Model file for the job. Use its own axes, mm. Face numbers are marked on the shaded views. A direction names the side the tool comes from. Give positions to 0.01 mm unless a question says otherwise; leave off trailing zeros. Loops run counter-clockwise (first coordinate to the right, second up) from the corner with the lowest first, then second, coordinate; pieces in that order, holes last. Notation, with made-up numbers: (68, -18) - (84, -18) arc R23 ccw to (84, -6) - close; hole circle Ø3 at (-38, 10.5). An arc over 180 degrees is marked (long way). Answer as CSV lines item,"result". Start each with the question number.
Item 1: Tool access for the marked faces 4, 5 and 6: list every direction of +Z, -Z, +X, -X, +Y, -Y with a clear straight run to the whole face (end or side of a thin tool).
Item 2: Pin check, flat tips, straight feed: pin 1 (8 mm diameter, centred on y = 4, z = 10.5, fed in from +X); pin 2 (3.5 mm diameter, centred on y = 2.5, z = 11.5, fed in from -X); pin 3 (3 mm diameter, centred on x = -16.5, y = 0.5, fed in from +Z). Stop position of each tip, or through.
Item 3: Pull direction X, two halves, no side cores. Call the marked faces 1, 2 and 3: pulls with the +X half, pulls with the -X half, needs draft (parallel to the pull), parting line crosses it, or undercut.
Item 4: Saw through at C-C on z = -14.5. Give the cut face in (x, y).
Item 5: Saw through at B-B on y = -4. Give the cut face in (x, z), plus the area to 3 significant figures.
Item 6: Drill centre lines: L1, parallel to X at y = 3.75, z = 0; L2, parallel to X at y = 5.5, z = 13; L3, parallel to X at y = -6, z = -18.5. Where is each one in solid material? Low to high. Write a range as from..to.
Item 7: Saw through at D-D on x = -19. Give the cut face in (y, z).
Item 8: Saw through at A-A on z = 0. Give the cut face in (x, y), plus the area to 3 significant figures.
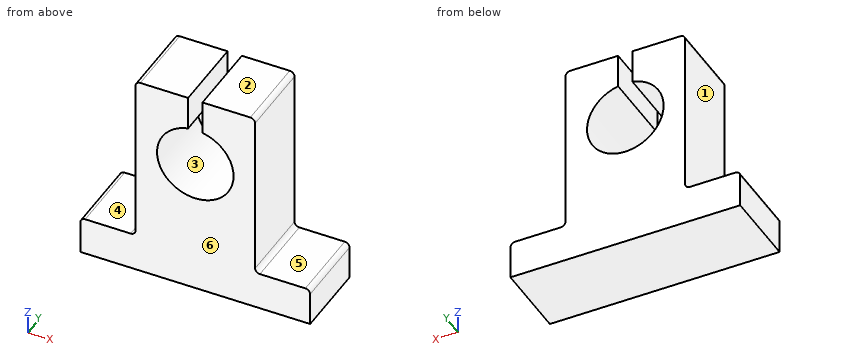
from build123d import *

# Parameters (mm, degrees)
F1_DEPTH = 8


with BuildPart() as f1:
    # F0 (on Front) → F1 (new body, symmetric)
    with BuildSketch(Plane.XZ):
        with BuildLine():
            Line((-24, -29), (24, -29))
            Line((24, -29), (24, -22))
            ThreePointArc((24, -22), (23.707107, -21.292893), (23, -21))
            Line((23, -21), (13.5, -21))
            ThreePointArc((13.5, -21), (12.792893, -20.707107), (12.5, -20))
            Line((12.5, -20), (12.5, 14))
            ThreePointArc((12.5, 14), (12.207107, 14.707107), (11.5, 15))
            Line((11.5, 15), (1.5, 15))
            Line((1.5, 15), (1.5, 7.858117))
            ThreePointArc((1.5, 7.858117), (0, -8), (-1.5, 7.858117))
            Line((-1.5, 7.858117), (-1.5, 15))
            Line((-1.5, 15), (-11.5, 15))
            ThreePointArc((-11.5, 15), (-12.207107, 14.707107), (-12.5, 14))
            Line((-12.5, 14), (-12.5, -20))
            ThreePointArc((-12.5, -20), (-12.792893, -20.707107), (-13.5, -21))
            Line((-13.5, -21), (-23, -21))
            ThreePointArc((-23, -21), (-23.707107, -21.292893), (-24, -22))
            Line((-24, -22), (-24, -29))
        make_face()
    extrude(amount=F1_DEPTH, both=True)


solid = f1.part
Responses:
1,face 4,"+Z, -X, +Y, -Y"
1,face 5,"+Z, +X, +Y, -Y"
1,face 6,"+Z, -Z, +X, -X, -Y"
2,pin 1,"x = 12.5"
2,pin 2,"x = -12.5"
2,pin 3,"z = -21"
3,face 1,"pulls with the -X half"
3,face 2,"needs draft"
3,face 3,"undercut"
4,outline,"(-12.5, -8) - (12.5, -8) - (12.5, 8) - (-12.5, 8) - close"
5,outline,"(-24, -29) - (24, -29) - (24, -22) arc R1 ccw to (23, -21) - (13.5, -21) arc R1 cw to (12.5, -20) - (12.5, 14) arc R1 ccw to (11.5, 15) - (1.5, 15) - (1.5, 7.86) arc R8 cw (long way) to (-1.5, 7.86) - (-1.5, 15) - (-11.5, 15) arc R1 ccw to (-12.5, 14) - (-12.5, -20) arc R1 cw to (-13.5, -21) - (-23, -21) arc R1 ccw to (-24, -22) - close"
5,area,"1,060 mm2"
6,L1,"-12.5..-8, 8..12.5"
6,L2,"-12.5..-1.5, 1.5..12.5"
6,L3,"-12.5..12.5"
7,outline,"(-8, -29) - (8, -29) - (8, -21) - (-8, -21) - close"
8,outline,"(-12.5, -8) - (-8, -8) - (-8, 8) - (-12.5, 8) - close; (8, -8) - (12.5, -8) - (12.5, 8) - (8, 8) - close"
8,area,"144 mm2"
